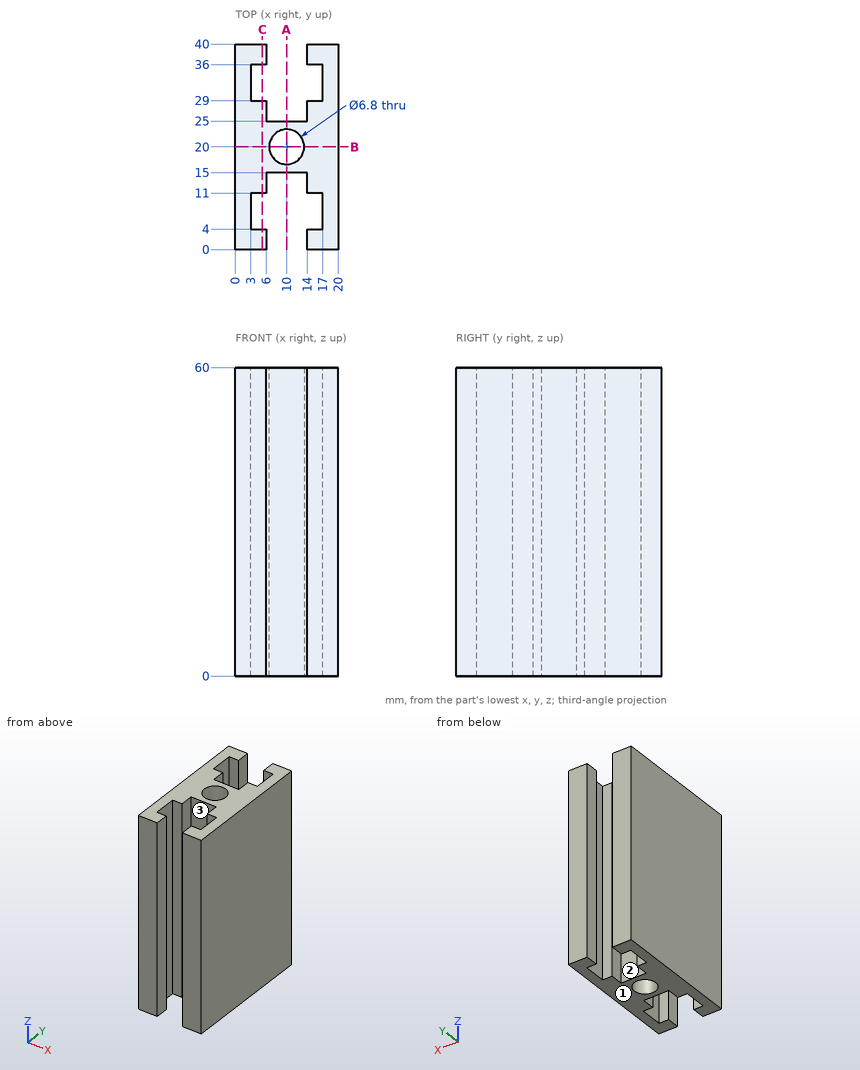
The figure shows three views and two pictorial views of one solid part (mm, origin at its lowest corner). Answer the questions. A direction names the side the tool comes from. Coordinates: 2 decimals unless noted, no trailing zeros. Write each loop counter-clockwise with the first axis right and the second up, starting at its lowest first coordinate (ties: lowest second). Pieces come first, ordered by that corner, then holes. Notation, with made-up numbers: (44.25, 14.25) -> (97.25, 14.25) arc R19 cw to (97.25, 27.25) -> close; hole circle Ø11 at (47.25, 61). An arc over 180 degrees is marked (long way). Return JSON: item names as keys, results as strings.
(1) Which of the six approach directions +Z, -Z, +X, -X, +Y, -Y give full straight-line access (tool end or side, diameter ignored) to the marked faces 1, 2 and 3?
Answers below:
{"face 1": "-Z, +X, -X, +Y, -Y", "face 2": "+Z, -Z, +Y", "face 3": "+Z, -Z, -Y"}
(2) The part is cut by section C-C on x = 5.25. Give the vertices of the cut face in (y, z).
Answers below:
{"outline": "(0, 0) -> (4, 0) -> (4, 60) -> (0, 60) -> close; (11, 0) -> (29, 0) -> (29, 60) -> (11, 60) -> close; (36, 0) -> (40, 0) -> (40, 60) -> (36, 60) -> close"}
(3) Consider line 1 along Y through (x, z) = (4.25, 43.5); line 2 along X through (y, z) = (20, 39); line 3 along Y through (x, z) = (10, 43.5). Determine where each line is inside the solid, lowest interval first. Write a range as from..to.
Answers below:
{"line 1": "0..4, 11..29, 36..40", "line 2": "0..6.6, 13.4..20", "line 3": "15..16.6, 23.4..25"}
(4) The part is cut by section B-B on y = 20. Give the vertices of the cut face in (x, z).
Answers below:
{"outline": "(0, 0) -> (6.6, 0) -> (6.6, 60) -> (0, 60) -> close; (13.4, 0) -> (20, 0) -> (20, 60) -> (13.4, 60) -> close"}
(5) The part is cut by section A-A on x = 10. Give the vertices of the cut face in (y, z), then the cut area to 3 significant figures.
Answers below:
{"outline": "(15, 0) -> (16.6, 0) -> (16.6, 60) -> (15, 60) -> close; (23.4, 0) -> (25, 0) -> (25, 60) -> (23.4, 60) -> close", "area": "192 mm^2"}
